Autodesk Inventor part; units mm, degrees
ref_plane "Work Plane1" through (88.9, -30.48, 0) normal (0, -1, 0) x (1, 0, 0)
ref_plane "YZ Plane" through (0, 0, 0) normal (1, 0, 0) x (0, 1, 0)
ref_plane "XZ Plane" through (0, 0, 0) normal (0, 1, 0) x (-1, 0, 0)
sketch "Sketch1" plane through (0, 0, 0) normal (0, 0, 1) x (1, 0, 0)
  line L0 (-88.9, -31.75) -> (88.9, -31.75)
  line L1 (88.9, -31.75) -> (88.9, 31.75)
  line L2 (88.9, 31.75) -> (-88.9, 31.75)
  line L3 (-88.9, 31.75) -> (-88.9, -31.75)
  line L4 (-88.9, -31.75) -> (88.9, 31.75) construction
  line L5 (88.9, -31.75) -> (-88.9, 31.75) construction
  point P0 (0, 0)
  dimension "d0" = 177.8
  dimension "d1" = 63.5
extrude "Extrusion1" add sketch "Sketch1" along normal blind 278
sketch "Sketch2" plane through (-88.9, 31.75, 0) normal (0, 1, 0) x (1, 0, 0)
  line L0 (177.8, -278) -> (0, -278)
  line L1 (177.8, 0) -> (0, 0)
  arc A0 (10.15, -263.3) -> (5.65, -263.3) centre (7.9, -263.3) ccw
  arc A1 (172.15, -263.3) -> (167.65, -263.3) centre (169.9, -263.3) ccw
  arc A2 (167.65, -27) -> (172.15, -27) centre (169.9, -27) ccw
  arc A3 (5.65, -27) -> (10.15, -27) centre (7.9, -27) ccw
  line L2 (7.9, -263.3) -> (7.9, -27) construction
  line L3 (7.9, -27) -> (169.9, -27) construction
  line L4 (169.9, -27) -> (169.9, -263.3) construction
  line L5 (7.9, -27) -> (7.9, 0) construction
  line L6 (7.9, -27) -> (0, 0) construction
  line L7 (169.9, -27) -> (177.8, 0) construction
  line L8 (167.65, -263.3) -> (167.65, -278)
  line L9 (172.15, -263.3) -> (172.15, -278)
  line L10 (5.65, -263.3) -> (5.65, -278)
  line L11 (10.15, -263.3) -> (10.15, -278)
  line L12 (10.15, -27) -> (10.15, 0)
  line L13 (5.65, -27) -> (5.65, 0)
  line L14 (172.15, -27) -> (172.15, 0)
  line L15 (167.65, -27) -> (167.65, 0)
  point P0 (88.9, 0)
  dimension "d4" = 2.25
  dimension "d5" = 236.3
  dimension "d6" = 162
  dimension "d14" = 27
extrude "Extrusion2" cut sketch "Sketch2" against normal up to surface (63.5 mm away)
ref_plane "Work Plane1" through (88.9, -30.48, 0) normal (0, -1, 0) x (1, 0, 0)
sketch "Sketch3" plane through (-88.9, 31.75, 278) normal (0, 1, 0) x (1, 0, 0)
  line L0 (0, 278) -> (0, 0)
  line L1 (177.8, 278) -> (177.8, 0)
  line L2 (176.53, 0) -> (176.53, 25.4)
  line L3 (176.53, 25.4) -> (1.27, 25.4)
  line L4 (1.27, 25.4) -> (1.27, 0)
  line L5 (1.27, 0) -> (176.53, 0)
  line L6 (1.27, 0) -> (0, 0) construction
  line L7 (177.8, 0) -> (176.53, 0) construction
  line L8 (1.27, 252.6) -> (176.53, 252.6)
  line L9 (176.53, 252.6) -> (176.53, 278)
  line L10 (176.53, 278) -> (1.27, 278)
  line L11 (1.27, 278) -> (1.27, 252.6)
  line L12 (1.27, 278) -> (0, 278) construction
  point P0 (88.9, 278)
  dimension "d9" = 1.27
  dimension "d10" = 25.4
extrude "Extrusion3" cut sketch "Sketch3" against normal up to surface (62.23 mm away)
properties part number "UHP-1500-230"
For this review, take the finished solid that the model builds, in its own axes (mm). A direction names the side the tool comes from. Round coordinates to 2 decimals unless told otherwise and drop trailing zeros. Loops run counter-clockwise (first coordinate to the right, second up) from the corner with the lowest first, then second, coordinate; pieces in that order, holes last. Notation, with made-up numbers: (-14, 68) - (0, 68) arc R12 ccw to (0, 88) - close; hole circle Ø3 at (71, -28.5). An arc over 180 degrees is marked (long way). Put each result on its own line as item: value. Start each with the question number.
1. Mouldability with a two-part tool opening along X and no side actions: class faces 1 (the flat face through (-83.25, 0.1, 26.6)), 2 (the flat face through (88, 0, 278)), 3 (the flat face through (83.25, 0.1, 26.6)), 4 (the flat face through (88.9, 0, 137)) as +X half, -X half, draft (parallel to the pull), parting line (faces both ways), or undercut.
2. Insertion check: P1, Ø3, axis at x = -53, y = 23, coming from the +Z side; P2, Ø20.5, axis at x = -34, z = 270.5, coming from the +Y side; P3, Ø6, axis at x = -62, y = 19, coming from the -Z side. Each pin has a flat end and moves straight along its axis. Give the tip position at first contact, or say it passes through.
3. Consider section B-B on x = 74. State the section outline as (y, z) points.
4. For faces 5 (the flat face through (-78.75, 0.1, 26.6)), 6 (the flat face through (-1, -31.75, 137)), 7 (the flat face through (-88.9, 0, 137)), 8 (the flat face through (87.63, 1, 13)), 9 (the flat face through (87.63, 1, 265)), list the 3-axis set-ups (+Z, -Z, +X, -X, +Y, -Y) from which the entire face can be reached by the end or side of a thin tool; tool diameter is ignored.
5. For probe 1 along X at (y, z) = (-16.5, 25); probe 2 along Z at (x, y) = (-42, 19); probe 3 along Y at (x, z) = (-63, 262.5), list the stretches that pass through material, from the lowest coordinate up. Write a range as [from, to].
6. Consider section C-C on y = -25. State the section outline as (x, z) points.
7. Consider section A-A on z = 21.5. State the section outline as (x, y) points, plus the area to 3 significant figures.
Result sheet:
1. face 1: undercut
1. face 2: draft
1. face 3: undercut
1. face 4: +X half
2. P1: z = 252.6
2. P2: y = -30.48
2. P3: z = 25.4
3. outline: (-31.75, 0) - (-30.48, 0) - (-30.48, 25.4) - (31.75, 25.4) - (31.75, 252.6) - (-30.48, 252.6) - (-30.48, 278) - (-31.75, 278) - close
4. face 5: -Z, +Y, -Y
4. face 6: +Z, -Z, +X, -X, -Y
4. face 7: +Z, -Z, -X, +Y, -Y
4. face 8: -Z, +Y
4. face 9: +Z, +Y
5. probe 1: [-88.9, -87.63], [87.63, 88.9]
5. probe 2: [25.4, 252.6]
5. probe 3: [-31.75, -30.48]
6. outline: (-88.9, 0) - (-87.63, 0) - (-87.63, 25.4) - (-83.25, 25.4) - (-83.25, 27) arc R2.25 cw to (-78.75, 27) - (-78.75, 25.4) - (78.75, 25.4) - (78.75, 27) arc R2.25 cw to (83.25, 27) - (83.25, 25.4) - (87.63, 25.4) - (87.63, 0) - (88.9, 0) - (88.9, 278) - (87.63, 278) - (87.63, 252.6) - (-87.63, 252.6) - (-87.63, 278) - (-88.9, 278) - close
7. outline: (-88.9, -31.75) - (-83.25, -31.75) - (-83.25, -30.48) - (-87.63, -30.48) - (-87.63, 31.75) - (-88.9, 31.75) - close; (-78.75, -31.75) - (78.75, -31.75) - (78.75, -30.48) - (-78.75, -30.48) - close; (83.25, -31.75) - (88.9, -31.75) - (88.9, 31.75) - (87.63, 31.75) - (87.63, -30.48) - (83.25, -30.48) - close
7. area: 372 mm^2
